The listing builds one solid part. Answer for the finished solid, in the listing's coordinates (mm). Give positions to 0.01 mm unless a question says otherwise; leave off trailing zeros. Write each loop counter-clockwise with the first axis right and the second up, starting at its lowest first coordinate (ties: lowest second). Pieces come first, ordered by that corner, then holes. Notation, with made-up numbers: (-9.5, -4) - (5.5, -4) arc R8 cw to (5.5, 3) - close; hole circle Ø3 at (86, 74.25). An arc over 180 degrees is marked (long way). Return JSON: item names as keys, results as strings.
from build123d import *

# Parameters (mm, degrees)
F2_R     = 10
F4_R     = 9
F6_W     = 85.2154158056
F6_H     = 10.0725549273
F7_DEPTH = 60


with BuildPart() as f3:
    # F3: sweep along a path in F0
    with BuildLine(Plane.XZ) as f3_path:
        Line((30, 58.5), (30, 0))
        ThreePointArc((30, 0), (0, -30), (-30, 0))
        Line((-30, 0), (-30, 24.9))
    # F2 (on line) → F3 (sweep)
    with BuildSketch(Plane(origin=(0, 0, 58.5), x_dir=(1, 0, 0), z_dir=(0, 0, -1))):
        with Locations((30, 0)):
            Circle(F2_R)
    sweep(path=f3_path.line)

    # F5: sweep along a path in F0
    with BuildLine(Plane.XZ) as f5_path:
        Line((-30, 24.9), (-30, 0))
        ThreePointArc((-30, 0), (0, -30), (30, 0))
        Line((30, 0), (30, 58.5))
    # F4 (on face) → F5 (sweep, cut)
    with BuildSketch(Plane.XY.offset(58.5)):
        with Locations((30, 0)):
            Circle(F4_R)
    sweep(path=f5_path.line, mode=Mode.SUBTRACT)


with BuildPart() as f7:
    # F6 (on Top) → F7 (new body, symmetric)
    with BuildSketch(Plane.XY):
        with Locations((-1.6176421195, -9.2803204898)):
            Rectangle(F6_W, F6_H)
    extrude(amount=F7_DEPTH, both=True)


with BuildPart() as f3_1:
    add(f3.part)

    # F8: cut F7
    add(f7.part, mode=Mode.SUBTRACT)


solid = f3_1.part
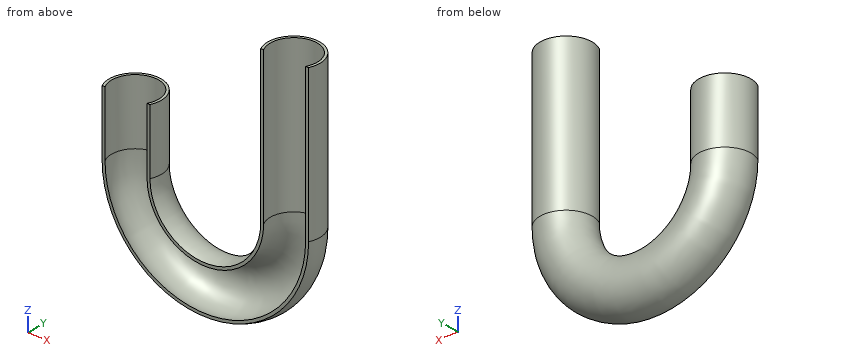
Item 1: Consider L1, parallel to X at y = 0, z = 20.5; L2, parallel to X at y = 0, z = 34; L3, parallel to X at y = -1, z = -8.5. Determine where each line is inside the solid, lowest interval first.
Answer below:
{"L1": "x = -40 to -39, -21 to -20, 20 to 21, 39 to 40", "L2": "x = 20 to 21, 39 to 40", "L3": "x = -39.04 to -38.01, -19.26 to -18.16, 18.16 to 19.26, 38.01 to 39.04"}
Item 2: A cutting plane is placed at B-B on z = 14. Determine the outline of the cut face in (x, y).
Answer below:
{"outline": "(-39.05, -4.24) - (-37.94, -4.24) arc R9 cw (long way) to (-22.06, -4.24) - (-20.95, -4.24) arc R10 ccw (long way) to start; (20.95, -4.24) - (22.06, -4.24) arc R9 cw (long way) to (37.94, -4.24) - (39.05, -4.24) arc R10 ccw (long way) to start"}
Item 3: A cutting plane is placed at A-A on y = 0. Determine the outline of the cut face in (x, z).
Answer below:
{"outline": "(-40, 0) arc R40 ccw to (40, 0) - (40, 58.5) - (39, 58.5) - (39, 0) arc R39 cw to (-39, 0) - (-39, 24.9) - (-40, 24.9) - close; (-21, 0) arc R21 ccw to (21, 0) - (21, 58.5) - (20, 58.5) - (20, 0) arc R20 cw to (-20, 0) - (-20, 24.9) - (-21, 24.9) - close"}
Item 4: Flat-ended cylindrical pins translate along their axes: P1, Ø5, axis at x = -28.5, y = -0.5, coming from the -Z side; P2, Ø1.5, axis at x = 31, z = -18.5, coming from the -Y side; P3, Ø1, axis at x = 5.5, y = 5, coming from the -Z side. Find the tip coordinate at first contact, or state that the pin passes through.
Answer below:
{"P1": "stops at z = -30.39", "P2": "stops at y = 5.84", "P3": "stops at z = -38.55"}
Item 5: A cutting plane is placed at C-C on y = 5.75. Determine the outline of the cut face in (x, z), then the cut area to 3 significant figures.
Answer below:
{"outline": "(-38.18, 0) arc R38.18 ccw to (38.18, 0) - (38.18, 58.5) - (36.92, 58.5) - (36.92, 0) arc R36.92 cw to (-36.92, 0) - (-36.92, 24.9) - (-38.18, 24.9) - close; (-23.08, 0) arc R23.08 ccw to (23.08, 0) - (23.08, 58.5) - (21.82, 58.5) - (21.82, 0) arc R21.82 cw to (-21.82, 0) - (-21.82, 24.9) - (-23.08, 24.9) - close", "area": "447 mm²"}
Item 6: A cutting plane is placed at D-D on z = 28.5. Determine the outline of the cut face in (x, y).
Answer below:
{"outline": "(20.95, -4.24) - (22.06, -4.24) arc R9 cw (long way) to (37.94, -4.24) - (39.05, -4.24) arc R10 ccw (long way) to start"}
